Source: CAD feature listing. Evaluate the final solid. Frame: model axes, mm. Give positions to 0.01 mm unless a question says otherwise; leave off trailing zeros. Order: outer loops, then holes, each group sorted by start corner. A loop starts at its lowest first (then second) coordinate and runs counter-clockwise, first axis right, second up. Notation, with made-up numbers: (-25, 33) - (-3, 33) arc R22 cw to (-3, 58) - close; hole circle Ø10 at (-16, 41). An arc over 180 degrees is marked (long way). Write each question's results on one line, items separated by ' | '. Start each with the question number.
Item 1: Contact query for flat-ended pins moving along their axis: pin 1 Ø3 at (x, z) = (0.5, -10) entering from -Y; pin 2 Ø6 at (x, z) = (2, 0) entering from +Y. Output: stop coordinate, or through.
Item 2: Section C-C on y = -2.7. Output: boundary loops of the cut face in (x, z).
Item 3: Section A-A on z = 18. Output: boundary loops of the cut face in (x, y), and give its area (3 significant figures).
Item 4: Section D-D on x = -2.5. Output: boundary loops of the cut face in (y, z), and give its area (3 significant figures).
Item 5: Section B-B on x = 0. Output: boundary loops of the cut face in (y, z).
Item 6: Line query: line 1 along Z through (x, y) = (0, -2.15); line 2 along X through (y, z) = (-2.35, -24); line 3 along Z through (x, y) = (-0.5, -2.2). Output: solid intervals per line, ascending.
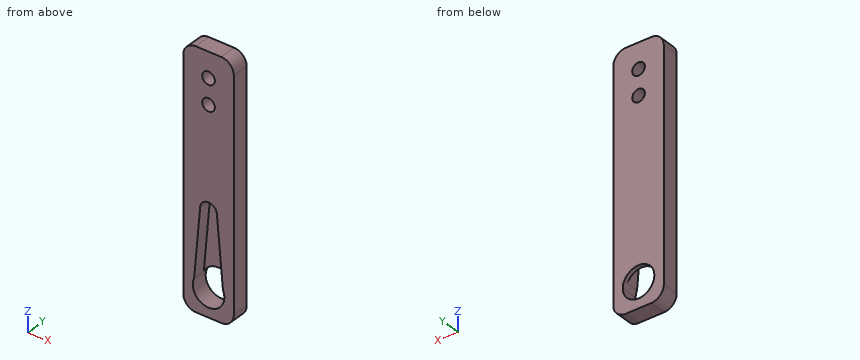
```python
from build123d import *

# Parameters (mm, degrees)
F0_R     = 1.5
F1_DEPTH = 4
F2_DEPTH = 1


with BuildPart() as f1:
    # F0 (on Front) → F1 (new body)
    with BuildSketch(Plane.XZ):
        with BuildLine():
            Line((-3, -30), (3, -30))
            ThreePointArc((3, -30), (5.12132, -29.12132), (6, -27))
            Line((6, -27), (6, 27))
            ThreePointArc((6, 27), (5.12132, 29.12132), (3, 30))
            Line((3, 30), (-3, 30))
            ThreePointArc((-3, 30), (-5.12132, 29.12132), (-6, 27))
            Line((-6, 27), (-6, -27))
            ThreePointArc((-6, -27), (-5.12132, -29.12132), (-3, -30))
        make_face()
        with BuildLine():
            ThreePointArc((3.75, -24), (-0.784385, -27.667048), (-3.421861, -22.465932))
            Line((-3.421861, -22.465932), (-2, -6))
            ThreePointArc((-2, -6), (0, -4), (2, -6))
            Line((2, -6), (3.421861, -22.465932))
            ThreePointArc((3.421861, -22.465932), (3.667048, -23.215615), (3.75, -24))
        make_face(mode=Mode.SUBTRACT)
        with Locations((0, 18)):
            Circle(F0_R, mode=Mode.SUBTRACT)
        with Locations((0, 24)):
            Circle(F0_R, mode=Mode.SUBTRACT)
    extrude(amount=F1_DEPTH)

    # F0 (on Front) → F2 (join)
    with BuildSketch(Plane.XZ):
        with BuildLine():
            Line((-2, -6), (-3.421861, -22.465932))
            ThreePointArc((-3.421861, -22.465932), (0, -20.25), (3.421861, -22.465932))
            Line((3.421861, -22.465932), (2, -6))
            ThreePointArc((2, -6), (0, -4), (-2, -6))
        make_face()
    extrude(amount=F2_DEPTH)


solid = f1.part
```
Evaluation:
1) pin 1: stops at y = -1 | pin 2: stops at y = 0
2) outline: (-6, -27) arc R3 ccw to (-3, -30) - (3, -30) arc R3 ccw to (6, -27) - (6, 27) arc R3 ccw to (3, 30) - (-3, 30) arc R3 ccw to (-6, 27) - close; hole (-3.42, -22.47) arc R3.75 ccw (long way) to (3.75, -24) arc R3.75 ccw to (3.42, -22.47) - (2, -6) arc R2 ccw to (-2, -6) - close; hole circle Ø3 at (0, 18); hole circle Ø3 at (0, 24)
3) outline: (-6, -4) - (-1.5, -4) - (-1.5, 0) - (-6, 0) - close; (1.5, -4) - (6, -4) - (6, 0) - (1.5, 0) - close | area: 36.0 mm^2
4) outline: (-4, -30) - (0, -30) - (0, -26.8) - (-4, -26.8) - close; (-4, -11.79) - (-1, -11.79) - (-1, -21.2) - (0, -21.2) - (0, 30) - (-4, 30) - close | area: 189 mm^2
5) outline: (-4, -30) - (0, -30) - (0, -27.75) - (-4, -27.75) - close; (-4, -4) - (-1, -4) - (-1, -20.25) - (0, -20.25) - (0, 16.5) - (-4, 16.5) - close; (-4, 19.5) - (0, 19.5) - (0, 22.5) - (-4, 22.5) - close; (-4, 25.5) - (0, 25.5) - (0, 30) - (-4, 30) - close
6) line 1: z = -30 to -27.75, -4 to 16.5, 19.5 to 22.5, 25.5 to 30 | line 2: x = -6 to -3.75, 3.75 to 6 | line 3: z = -30 to -27.72, -4.06 to 16.59, 19.41 to 22.59, 25.41 to 30
